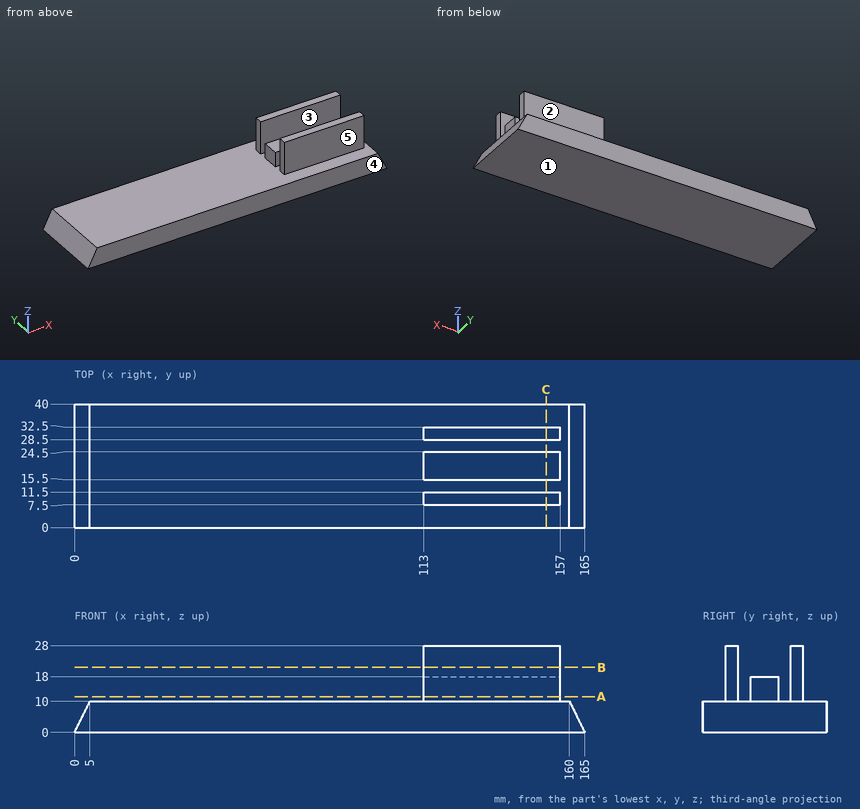
Can you work these out from the drawing? Everything is in mm from the part's minimum corner. A direction names the side the tool comes from. Give positions to 0.01 mm unless a question says otherwise; leave off trailing zeros. Loops run counter-clockwise (first coordinate to the right, second up) from the corner with the lowest first, then second, coordinate; pieces in that order, holes last. Notation, with made-up numbers: (-21, 35) - (-2, 35) arc R16 ccw to (-2, 45) - close; hole circle Ø11 at (-13.5, -19.5). An arc over 180 degrees is marked (long way). Use one line per item in the form item = value.
1. I'm going to push flat-ended pins straight in: pin 1 Ø10 at (x, y) = (58, 27) entering from +Z; pin 2 Ø1.5 at (y, z) = (9.5, 23.5) entering from -X; pin 3 Ø1.5 at (y, z) = (5, 4) entering from -X (3 decimals). Where does each tip first touch, or does it pass through?
Response values:
pin_1 = 10
pin_2 = 113
pin_3 = 1.625
2. I need wall thicknesses on probe 1 along Z at (x, y) = (53, 38); probe 2 along Y at (x, z) = (154.5, 20); probe 3 along X at (y, z) = (20, 12.5). Which ranges of each line are inside material? Lowest first, please.
Response values:
probe_1 = 0 to 10
probe_2 = 7.5 to 11.5, 28.5 to 32.5
probe_3 = 113 to 157
3. I want a section at A-A (z = 11.5). Please give me the cut outline in (x, y).
Response values:
outline = (113, 7.5) - (157, 7.5) - (157, 11.5) - (113, 11.5) - close; (113, 15.5) - (157, 15.5) - (157, 24.5) - (113, 24.5) - close; (113, 28.5) - (157, 28.5) - (157, 32.5) - (113, 32.5) - close
4. Thinking about a two-plate mould opening in Y: for the marked faces 1, 2 and 3, which applies, released by +Y, released by -Y, zero draft, split by the parting line, or undercut?
Response values:
face_1 = zero draft
face_2 = released by +Y
face_3 = undercut
5. I want a section at B-B (z = 21). Please give me the cut outline in (x, y).
Response values:
outline = (113, 7.5) - (157, 7.5) - (157, 11.5) - (113, 11.5) - close; (113, 28.5) - (157, 28.5) - (157, 32.5) - (113, 32.5) - close
6. On a 3-axis mill with a long thin cutter (end or side, diameter ignored), from which of +Z, -Z, +X, -X, +Y, -Y can I reach the whole of each face in a straight line? I mean the marked faces 4 and 5. Say none if no direction works.
Response values:
face_4 = +Z, -Z, +X, -X, -Y
face_5 = +Z, +X, -X, -Y
7. I want a section at C-C (x = 152.5). Please give me the cut outline in (y, z).
Response values:
outline = (0, 0) - (40, 0) - (40, 10) - (32.5, 10) - (32.5, 28) - (28.5, 28) - (28.5, 10) - (24.5, 10) - (24.5, 18) - (15.5, 18) - (15.5, 10) - (11.5, 10) - (11.5, 28) - (7.5, 28) - (7.5, 10) - (0, 10) - close
